from build123d import *

# Parameters (mm, degrees)
CROQUIS1_R              = 25
SALIENTE_EXTRUIR1_DEPTH = 2.8
CROQUIS2_W              = 2.75
CROQUIS2_H              = 18
CORTAR_EXTRUIR1_DEPTH   = 3.8
MATRIZC2_COUNT          = 3
MATRIZC2_ANGLE          = 233.12


with BuildPart() as part:
    # Croquis1 → Saliente-Extruir1 (new body)
    with BuildSketch(Plane.XY):
        Circle(CROQUIS1_R)
    extrude(amount=SALIENTE_EXTRUIR1_DEPTH)

    # Croquis2 → Cortar-Extruir1 (cut, through all)
    with BuildSketch(Plane.XY):
        with Locations((0, 25)):
            Rectangle(CROQUIS2_W, CROQUIS2_H)
    cortar_extruir1 = extrude(amount=CORTAR_EXTRUIR1_DEPTH, mode=Mode.SUBTRACT)

    # MatrizC2: Cortar-Extruir1 ×3 about axis
    matrizc2_axis = Axis((0, 0, 0), (0, 0, 1))
    for i in range(1, MATRIZC2_COUNT):
        add(cortar_extruir1.rotate(matrizc2_axis, i * MATRIZC2_ANGLE / (MATRIZC2_COUNT - 1)), mode=Mode.SUBTRACT)


solid = part.part
The listing builds one solid part. Answer for the finished solid, in the listing's coordinates (mm). A direction names the side the tool comes from. Give positions to 0.01 mm unless a question says otherwise; leave off trailing zeros. Write each loop counter-clockwise with the first axis right and the second up, starting at its lowest first coordinate (ties: lowest second). Pieces come first, ordered by that corner, then holes. Notation, with made-up numbers: (-14.75, -5) -> (-9.75, -5) arc R15 ccw to (-9.75, -1) -> close; hole circle Ø6 at (-26, -7.75). An arc over 180 degrees is marked (long way). Use a Markdown table: item, result.
(1) Section A-A, the plane z = 0.85 is taken. Determine the outline of the cut face in (x, y) (1 decimal).
Return value:
| item | result |
|---|---|
| outline | (-22.9, -9.9) -> (-14.9, -5.9) -> (-13.7, -8.4) -> (-21.7, -12.4) arc R25 ccw to (19.1, -16.1) -> (12, -10.7) -> (13.6, -8.5) -> (20.8, -13.9) arc R25 ccw to (1.4, 25) -> (1.4, 16) -> (-1.4, 16) -> (-1.4, 25) arc R25 ccw to start |
(2) Flat-ended cylindrical pins translate along their axes: P1, Ø1, axis at x = 13.5, z = 0.5, coming from the +Y side; P2, Ø1.4, axis at y = 21, z = 1, coming from the +X side; P3, Ø1, axis at y = -18, z = 0.5, coming from the +X side. Find the tip coordinate at first contact, or state that the pin passes through.
Return value:
| item | result |
|---|---|
| P1 | y = 21.35 |
| P2 | x = 14.59 |
| P3 | x = 17.85 |
(3) For faces 5 (the flat face through (12.8, -9.6, 1.4)), 6 (the flat face through (1.375, 20, 1)), 7 (the cylindrical face through (-21.087, 13.429, 1.38)), determine the directions among +Z, -Z, +X, -X, +Y, -Y from which every point of the face is accessible in a straight line to the end or side of a thin tool.
Return value:
| item | result |
|---|---|
| face 5 | +Z, -Z |
| face 6 | +Z, -Z, +Y |
| face 7 | +Z, -Z, -X |
(4) Find the intervals of material crossed by probe 1 along X at (y, z) = (0, 2.65); probe 2 along X at (y, z) = (20, 0.25) (3 decimals); probe 3 along Y at (x, z) = (-17.5, 2.4), in increasing order. Write a range as from..to.
Return value:
| item | result |
|---|---|
| probe 1 | -25..25 |
| probe 2 | -15..-1.375, 1.375..15 |
| probe 3 | -17.85..-10.29, -7.21..17.85 |
(5) Determine the mould class of faces 1 (the flat face through (0, 0, 0)), 2 (the flat face through (15.507, -13.354, 1.38)), 3 (the flat face through (17.158, -11.154, 1.38)), 4 (the cylindrical face through (22.524, 10.848, 1.38)) for opening direction X: released by +X, released by -X, zero draft, split by the parting line, or undercut.
Return value:
| item | result |
|---|---|
| face 1 | zero draft |
| face 2 | undercut |
| face 3 | undercut |
| face 4 | released by +X |
(6) Section D-D, the plane y = -20 is taken. Determine the outline of the cut face in (x, z), then the cut area to 3 significant figures.
Return value:
| item | result |
|---|---|
| outline | (-15, 0) -> (15, 0) -> (15, 2.8) -> (-15, 2.8) -> close |
| area | 84.0 mm2 |
(7) Section C-C, the plane y = 21 is taken. Determine the outline of the cut face in (x, z) (3 decimals), then the cut area to 3 significant figures.
Return value:
| item | result |
|---|---|
| outline | (-13.565, 0) -> (-1.375, 0) -> (-1.375, 2.8) -> (-13.565, 2.8) -> close; (1.375, 0) -> (13.565, 0) -> (13.565, 2.8) -> (1.375, 2.8) -> close |
| area | 68.3 mm2 |
(8) Section B-B, the plane x = -18.5 is taken. Determine the outline of the cut face in (y, z).
Return value:
| item | result |
|---|---|
| outline | (-16.82, 0) -> (-10.79, 0) -> (-10.79, 2.8) -> (-16.82, 2.8) -> close; (-7.71, 0) -> (16.82, 0) -> (16.82, 2.8) -> (-7.71, 2.8) -> close |
